The listing builds one solid part. Answer for the finished solid, in the listing's coordinates (mm). Face numbers are marked on the shaded views. A direction names the side the tool comes from. Give positions to 0.01 mm unless a question says otherwise; leave off trailing zeros. Write each loop counter-clockwise with the first axis right and the second up, starting at its lowest first coordinate (ties: lowest second). Pieces come first, ordered by that corner, then holes. Notation, with made-up numbers: (11.5, 4.5) - (19.5, 4.5) arc R12 cw to (19.5, 27.5) - close; hole circle Ø10 at (-37.75, -11.5). An arc over 180 degrees is marked (long way). Answer in a Markdown table with one row per item. Add a question column.
from build123d import *

# Parameters (mm, degrees)
BEARINGSKE_R   = 4
BEARINGSKE_R_2 = 2.5
BEARING_DEPTH  = 2.5
FLANGE_START   = -0.6
FLANGESKE_R    = 4.6
FLANGESKE_R_2  = 4
FLANGE_DEPTH   = 0.6
CHAMFER_2_SIZE = 0.1


with BuildPart() as part:
    # BearingSke → Bearing (new body)
    with BuildSketch(Plane.XY):
        Circle(BEARINGSKE_R)
        Circle(BEARINGSKE_R_2, mode=Mode.SUBTRACT)
    extrude(amount=BEARING_DEPTH)

    # FlangeSke → Flange (add)
    with BuildSketch(Plane.XY.offset(2.5).offset(FLANGE_START)):
        Circle(FLANGESKE_R)
        Circle(FLANGESKE_R_2, mode=Mode.SUBTRACT)
    extrude(amount=FLANGE_DEPTH)

    # Chamfer 2
    chamfer_2_edges = [part.edges().sort_by_distance(p)[0] for p in [
        (-4.6, 0, 1.9),
        (-4.6, 0, 2.5),
        (-4, 0, 0),
        (-2.5, 0, 0),
        (-2.5, 0, 2.5),
    ]]
    chamfer(chamfer_2_edges, length=CHAMFER_2_SIZE)


solid = part.part
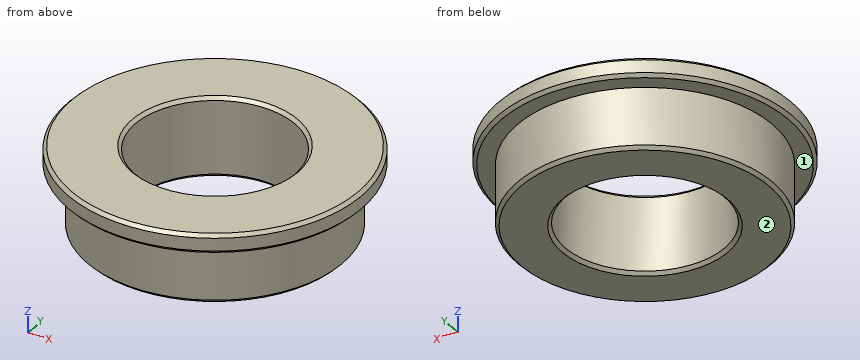
1. Section C-C (z = 0.3) is taken. Give the vertices of the cut face in (x, y).
2. Section A-A (x = 0) is taken. Give the vertices of the cut face in (y, z), and give its area (3 significant figures).
3. Straight lines are drawn through the part: L1, parallel to Y at x = 0, z = 0.8; L2, parallel to Z at x = 3.5, y = 2.75; L3, parallel to Y at x = -1.5, z = 2.05. For each, find the intervals that lie inside material, in ascending order. Write a range as [from, to].
4. A tool of negligible diameter and unlimited length cuts with its end or side. For the marked faces 1 and 2, from which of +Z, -Z, +X, -X, +Y, -Y can it reach the whole face along a straight path? Write none if from no direction.
5. Given pin 1 Ø1 at (x, z) = (-3, 0.5) entering from +Y; pin 2 Ø1.5 at (x, z) = (2, 1.5) entering from -Y; pin 3 Ø1 at (x, z) = (-3, 1.5) entering from -Y, each flat-ended and moving along its own axis, determine where each tip first touches the part or whether it passes through.
Geometry check:
| question | item | result |
|---|---|---|
| 1 | outline | circle Ø8 at (0, 0); hole circle Ø5 at (0, 0) |
| 2 | outline | (-4.6, 2) - (-4.5, 1.9) - (-4, 1.9) - (-4, 0.1) - (-3.9, 0) - (-2.6, 0) - (-2.5, 0.1) - (-2.5, 2.4) - (-2.6, 2.5) - (-4.5, 2.5) - (-4.6, 2.4) - close; (2.5, 0.1) - (2.6, 0) - (3.9, 0) - (4, 0.1) - (4, 1.9) - (4.5, 1.9) - (4.6, 2) - (4.6, 2.4) - (4.5, 2.5) - (2.6, 2.5) - (2.5, 2.4) - close |
| 2 | area | 8.17 mm² |
| 3 | L1 | [-4, -2.5], [2.5, 4] |
| 3 | L2 | [1.9, 2.5] |
| 3 | L3 | [-4.35, -2], [2, 4.35] |
| 4 | face 1 | -Z |
| 4 | face 2 | -Z, +X, -X, +Y, -Y |
| 5 | pin 1 | y = 3.12 |
| 5 | pin 2 | y = -4.37 |
| 5 | pin 3 | y = -3.6 |
